```python
from build123d import *

# Parameters (mm, degrees)
SKETCH1_R                       = 73.025
BASE_EXTRUDE_DEPTH              = 12.7
STANDOFFS_DEPTH                 = 31.75
CIRPATTERN1_COUNT               = 4
F_10_32_TAPPED_HOLE1_AT_2_COUNT = 2
F_10_32_TAPPED_HOLE1_AT_2_PITCH = 10
CIRPATTERN2_COUNT               = 4
SKETCH3_R                       = 15.875
SKETCH3_R_2                     = 1.905
SKETCH3_R_3                     = 4.99999
BODY_HOLES_DEPTH                = 12.7


with BuildPart() as part:
    # Sketch1 → Base Extrude (new body)
    with BuildSketch(Plane(origin=(0, 0, 0), x_dir=(1, 0, 0), z_dir=(0, 1, 0))):
        Circle(SKETCH1_R)
    extrude(amount=BASE_EXTRUDE_DEPTH)

    # Sketch2 → Standoffs (add)
    with BuildSketch(Plane(origin=(0, 12.7, 0), x_dir=(1, 0, 0), z_dir=(0, 1, 0))):
        with BuildLine():
            ThreePointArc((-65.454301807, -12.7), (-66.675, 0), (-65.454301807, 12.7))
            Line((-65.454301807, 12.7), (-71.688044836, 13.90952381))
            ThreePointArc((-71.688044836, 13.90952381), (-73.025, 0), (-71.688044836, -13.90952381))
            Line((-71.688044836, -13.90952381), (-65.454301807, -12.7))
        make_face()
    standoffs = extrude(amount=STANDOFFS_DEPTH)

    # CirPattern1: Standoffs ×4 about axis
    cirpattern1_axis = Axis((0, 0, 0), (0, 1, 0))
    for i in range(1, CIRPATTERN1_COUNT):
        add(standoffs.rotate(cirpattern1_axis, i * 360 / CIRPATTERN1_COUNT))

    # Sketch7 → #10-32 Tapped Hole1 (revolve, cut)
    with BuildSketch(Plane(origin=(-73.025, 39.45, 0), x_dir=(0, 0, 1), z_dir=(0, 1, 0))):
        Polygon((0, 0), (0, 26.613317848), (2.0193, 25.4), (2.0193, 0), align=None)
    f_10_32_tapped_hole1 = revolve(axis=Axis((-79.375, 39.45, 0), (1, 0, 0)), mode=Mode.SUBTRACT)

    # #10-32 Tapped Hole1 at 2: #10-32 Tapped Hole1 ×2
    with Locations(*[(0, -i * F_10_32_TAPPED_HOLE1_AT_2_PITCH, 0) for i in range(1, F_10_32_TAPPED_HOLE1_AT_2_COUNT)]):
        add(f_10_32_tapped_hole1, mode=Mode.SUBTRACT)

    # CirPattern2: #10-32 Tapped Hole1 ×4 about axis
    cirpattern2_axis = Axis((0, 0, 0), (0, 1, 0))
    for i in range(1, CIRPATTERN2_COUNT):
        add(f_10_32_tapped_hole1.rotate(cirpattern2_axis, i * 360 / CIRPATTERN2_COUNT), mode=Mode.SUBTRACT)

    # CirPattern2 copy 1 sketch → CirPattern2 copy 1 (revolve, cut)
    with BuildSketch(Plane(origin=(0, 29.45, 73.025), x_dir=(1, 0, 0), z_dir=(0, 1, 0))):
        Polygon((0, 0), (0, 26.613317848), (2.0193, 25.4), (2.0193, 0), align=None)
    revolve(axis=Axis((0, 29.45, 79.375), (0, 0, -1)), mode=Mode.SUBTRACT)

    # CirPattern2 copy 2 sketch → CirPattern2 copy 2 (revolve, cut)
    with BuildSketch(Plane(origin=(73.025, 29.45, 0), x_dir=(0, 0, -1), z_dir=(0, 1, 0))):
        Polygon((0, 0), (0, 26.613317848), (2.0193, 25.4), (2.0193, 0), align=None)
    revolve(axis=Axis((79.375, 29.45, 0), (-1, 0, 0)), mode=Mode.SUBTRACT)

    # CirPattern2 copy 3 sketch → CirPattern2 copy 3 (revolve, cut)
    with BuildSketch(Plane(origin=(0, 29.45, -73.025), x_dir=(-1, 0, 0), z_dir=(0, 1, 0))):
        Polygon((0, 0), (0, 26.613317848), (2.0193, 25.4), (2.0193, 0), align=None)
    revolve(axis=Axis((0, 29.45, -79.375), (0, 0, 1)), mode=Mode.SUBTRACT)

    # Sketch3 → Body-Holes (cut)
    with BuildSketch(Plane(origin=(0, 12.7, 0), x_dir=(1, 0, 0), z_dir=(0, 1, 0))):
        with Locations((-24.34209, 0)):
            Circle(SKETCH3_R)
        with Locations((24.34209, 0)):
            Circle(SKETCH3_R)
        with Locations((-24.34209, 19.05)):
            Circle(SKETCH3_R_2)
        with Locations((-24.34209, -19.05)):
            Circle(SKETCH3_R_2)
        with Locations((-17.37995, -44.45)):
            Circle(SKETCH3_R_3)
        with Locations((17.37995, -44.45)):
            Circle(SKETCH3_R_3)
        with Locations((17.37995, 44.45)):
            Circle(SKETCH3_R_3)
        with Locations((-17.37995, 44.45)):
            Circle(SKETCH3_R_3)
        with Locations((-43.39209, 0)):
            Circle(SKETCH3_R_2)
        with Locations((-5.29209, 0)):
            Circle(SKETCH3_R_2)
        with Locations((24.34209, -19.05)):
            Circle(SKETCH3_R_2)
        with Locations((43.39209, 0)):
            Circle(SKETCH3_R_2)
        with Locations((5.29209, 0)):
            Circle(SKETCH3_R_2)
        with Locations((24.34209, 19.05)):
            Circle(SKETCH3_R_2)
    extrude(amount=-BODY_HOLES_DEPTH, mode=Mode.SUBTRACT)


solid = part.part
```
Can you work these out from the model? Positions are in its coordinate system, mm. A direction names the side the tool comes from. Give positions to 0.01 mm unless a question says otherwise; leave off trailing zeros. Loops run counter-clockwise (first coordinate to the right, second up) from the corner with the lowest first, then second, coordinate; pieces in that order, holes last. Notation, with made-up numbers: M 28.5,49.5 L 64.5,49.5 A24 ccw 64.5,72.5 Z; hole C 25.25,-17.75 d11. An arc over 180 degrees is marked long. One line per question, with ' | ' between items. Start each with the question number.
Q1. If we mould it in two halves opening along Y, with no side actions, what happens to faces 5 (the flat face through (-13.313, 28.353, -68.615)), 6 (the flat face through (69, 44.45, 0)), 7 (the cylindrical face through (69.879, 31.241, -0.932)), 8 (the cylindrical face through (-0.263, 37.448, 69.879))? For each: +Y half, -Y half, draft (parallel to the pull), parting line (faces both ways), or undercut.
Q2. For pin 1 Ø6 at (x, z) = (5.29, 0) entering from +Y; pin 2 Ø3 at (x, y) = (11, 31.5) entering from -Z, each with a flat end and sliding along its axis, tell me the tip position at first contact or that it passes through.
Q3. If we section it at D-D (x = 18): Please give me the cut outline in (y, z).
Q4. If I drill on line 1 (Y direction, x = 0, z = 71); line 2 (X direction, y = 9.5, z = -44.45); line 3 (X direction, y = 5.5, z = -4.5), over which ranges is the centre line in solid material (lowest first)? Write a range as from..to.
Q5. If we section it at C-C (z = -19.05): Please give me the cut outline in (x, y).
Q6. If we section it at B-B (y = 23.5): Please give me the cut outline in (x, z) (3 decimals), plus the area to 3 significant figures.
Q7. If we section it at A-A (x = 0): Please give me the cut outline in (y, z) (3 decimals).
Q8. For faces 1 (the cylindrical face through (-66.62, 28.35, -2.66)), 2 (the flat face through (-68.528, 28.353, -13.296)), 3 (the flat face through (13.313, 28.353, 68.615)), 4 (the flat face through (-13.296, 28.353, 68.528)), which set-ups out of +Z, -Z, +X, -X, +Y, -Y let a thin tool reach every point of the face, with its end or its side?
Computed:
1) face 5: draft | face 6: +Y half | face 7: undercut | face 8: undercut
2) pin 1: stops at y = 12.7 | pin 2: stops at z = -72.4
3) outline: M 0,-70.77 L 12.7,-70.77 L 12.7,-49.41 L 0,-49.41 Z; M 0,-39.49 L 12.7,-39.49 L 12.7,-14.55 L 0,-14.55 Z; M 0,14.55 L 12.7,14.55 L 12.7,39.49 L 0,39.49 Z; M 0,49.41 L 12.7,49.41 L 12.7,70.77 L 0,70.77 Z
4) line 1: y = 0..27.43, 31.47..37.43, 41.47..44.45 | line 2: x = -57.94..-22.38, -12.38..12.38, 22.38..57.94 | line 3: x = -72.89..-39.57, -9.12..9.12, 39.57..72.89
5) outline: M -70.5,0 L -26.25,0 L -26.25,12.7 L -70.5,12.7 Z; M -22.44,0 L 22.44,0 L 22.44,12.7 L -22.44,12.7 Z; M 26.25,0 L 70.5,0 L 70.5,12.7 L 26.25,12.7 Z
6) outline: M -71.688,-13.91 L -65.454,-12.7 A66.675 cw -65.454,12.7 L -71.688,13.91 A73.025 ccw Z; M -13.91,-71.688 A73.025 ccw 13.91,-71.688 L 12.7,-65.454 A66.675 cw -12.7,-65.454 Z; M -13.91,71.688 L -12.7,65.454 A66.675 cw 12.7,65.454 L 13.91,71.688 A73.025 ccw Z; M 65.454,-12.7 L 71.688,-13.91 A73.025 ccw 71.688,13.91 L 65.454,12.7 A66.675 cw Z | area: 680 mm²
7) outline: M 0,-73.025 L 27.431,-73.025 L 27.431,-66.675 L 12.7,-66.675 L 12.7,66.675 L 27.431,66.675 L 27.431,73.025 L 0,73.025 Z; M 31.469,-73.025 L 37.431,-73.025 L 37.431,-66.675 L 31.469,-66.675 Z; M 31.469,66.675 L 37.431,66.675 L 37.431,73.025 L 31.469,73.025 Z; M 41.469,-73.025 L 44.45,-73.025 L 44.45,-66.675 L 41.469,-66.675 Z; M 41.469,66.675 L 44.45,66.675 L 44.45,73.025 L 41.469,73.025 Z
8) face 1: +Y | face 2: -Z, +Y | face 3: +X, +Y | face 4: -X, +Y
